from build123d import *

# Parameters (mm, degrees)
SKETCH_1_W             = 232
SKETCH_1_H             = 132
SKETCH_1_R             = 2.25
SM_BASE_FLANGE_1_DEPTH = 4
FILLET_1_R             = 16


# Sheet-metal steps are written as plain solids
with BuildPart() as part:
    # Sketch 1 → Базовая кромка1 (new body)
    with BuildSketch(Plane.XY):
        Rectangle(SKETCH_1_W, SKETCH_1_H)
        with Locations((0, 57.5)):
            Circle(SKETCH_1_R, mode=Mode.SUBTRACT)
        with Locations((-90, 57.5)):
            Circle(SKETCH_1_R, mode=Mode.SUBTRACT)
        with Locations((90, 57.5)):
            Circle(SKETCH_1_R, mode=Mode.SUBTRACT)
        with Locations((-107.5, 0)):
            Circle(SKETCH_1_R, mode=Mode.SUBTRACT)
        with Locations((107.5, 0)):
            Circle(SKETCH_1_R, mode=Mode.SUBTRACT)
        with Locations(Location((90, -57.5, 0), (0, 0, 180))):
            Circle(SKETCH_1_R, mode=Mode.SUBTRACT)
        with Locations(Location((0, -57.5, 0), (0, 0, 180))):
            Circle(SKETCH_1_R, mode=Mode.SUBTRACT)
        with Locations(Location((-90, -57.5, 0), (0, 0, 180))):
            Circle(SKETCH_1_R, mode=Mode.SUBTRACT)
    extrude(amount=-SM_BASE_FLANGE_1_DEPTH)

    # Скругление1
    fillet_1_edges = [part.edges().sort_by_distance(p)[0] for p in [
        (-116, 66, -2),
        (116, 66, -2),
        (116, -66, -2),
        (-116, -66, -2),
    ]]
    fillet(fillet_1_edges, radius=FILLET_1_R)


solid = part.part
Can you work these out from the model? Positions are in its coordinate system, mm. Coordinates: 2 decimals unless noted, no trailing zeros. Order: outer loops, then holes, each group sorted by start corner. A loop starts at its lowest first (then second) coordinate and runs counter-clockwise, first axis right, second up. Notation, with made-up numbers: M 84,71.5 L 94,71.5 A13 ccw 94,87.5 Z; hole C -35.75,34 d1. An arc over 180 degrees is marked long. Answer as CSV lines item,"result".
(1) Please list where these lines run through material, in increasing order: L1, parallel to Y at x = -90, z = -1; L2, parallel to X at y = 58.5, z = -1.1; L3, parallel to X at y = -57.5, z = -0.85.
Geometry check:
L1,"-66 to -59.75, -55.25 to 55.25, 59.75 to 66"
L2,"-113.56 to -92.02, -87.98 to -2.02, 2.02 to 87.98, 92.02 to 113.56"
L3,"-114.13 to -92.25, -87.75 to -2.25, 2.25 to 87.75, 92.25 to 114.13"
(2) Suppose I cut it at D-D on x = 107.5. Please give me the cut outline in (y, z).
Geometry check:
outline,"M -64.13,-4 L -2.25,-4 L -2.25,0 L -64.13,0 Z; M 2.25,-4 L 64.13,-4 L 64.13,0 L 2.25,0 Z"
(3) If we mould it in two halves opening along Y, with no side actions, what happens to faces 1 (the flat face through (-2, 1, -4)), 2 (the cylindrical face through (-111.437, -61.189, -2.028)), 3 (the cylindrical face through (-105.42, -0.86, -1.97))? For each: released by +Y, released by -Y, zero draft, split by the parting line, or undercut.
Geometry check:
face 1,"zero draft"
face 2,"released by -Y"
face 3,"undercut"
(4) Suppose I cut it at C-C on y = 57.5. Please give me the cut outline in (x, z).
Geometry check:
outline,"M -114.13,-4 L -92.25,-4 L -92.25,0 L -114.13,0 Z; M -87.75,-4 L -2.25,-4 L -2.25,0 L -87.75,0 Z; M 2.25,-4 L 87.75,-4 L 87.75,0 L 2.25,0 Z; M 92.25,-4 L 114.13,-4 L 114.13,0 L 92.25,0 Z"
(5) Suppose I cut it at B-B on x = 0. Please give me the cut outline in (y, z).
Geometry check:
outline,"M -66,-4 L -59.75,-4 L -59.75,0 L -66,0 Z; M -55.25,-4 L 55.25,-4 L 55.25,0 L -55.25,0 Z; M 59.75,-4 L 66,-4 L 66,0 L 59.75,0 Z"
(6) I'm going to push a flat-ended pin straight in: pin 1 (4 mm diameter, centred on x = 0, y = -57.5, fed in from -Z). Where does the tip first touch, or does it pass through?
Geometry check:
pin 1,"through"
(7) Suppose I cut it at A-A on y = 0. Please give me the cut outline in (x, z).
Geometry check:
outline,"M -116,-4 L -109.75,-4 L -109.75,0 L -116,0 Z; M -105.25,-4 L 105.25,-4 L 105.25,0 L -105.25,0 Z; M 109.75,-4 L 116,-4 L 116,0 L 109.75,0 Z"
